```python
from build123d import *

# Parameters (mm, degrees)
F0_R     = 104
F0_R_2   = 68.5
F1_DEPTH = 19
F2_R     = 80
F2_R_2   = 74.5
F3_DEPTH = 14.1
F4_R     = 80
F5_DEPTH = 12
F6_SIZE2 = 1.1547005384
F6_SIZE  = 2
F7_R     = 5
F9_D     = 14
F9_DEPTH = 25.5
F9_TIP   = 4.2060243332


with BuildPart() as f1:
    # F0 (on Right) → F1 (new body)
    with BuildSketch(Plane.YZ):
        Circle(F0_R)
        Circle(F0_R_2, mode=Mode.SUBTRACT)
    extrude(amount=-F1_DEPTH)

    # F2 (on face) → F3 (join)
    with BuildSketch(Plane.YZ):
        Circle(F2_R)
        Circle(F2_R_2, mode=Mode.SUBTRACT)
    extrude(amount=F3_DEPTH)

    # F4 (on face) → F5 (cut)
    with BuildSketch(Plane(origin=(-19, 0, 0), x_dir=(0, -1, 0), z_dir=(-1, 0, 0))):
        Circle(F4_R)
    extrude(amount=-F5_DEPTH, mode=Mode.SUBTRACT)

    # F6
    f6_edges = [f1.edges().sort_by_distance(p)[0] for p in [
        (14.1, -80, 0),
    ]]
    f6_side = f1.faces().sort_by_distance((7.05, -80, 0))[0]
    chamfer(f6_edges, length=F6_SIZE, length2=F6_SIZE2, reference=f6_side)

    # F7
    f7_edges = [f1.edges().sort_by_distance(p)[0] for p in [
        (0, -74.5, 0),
    ]]
    fillet(f7_edges, radius=F7_R)

    # F9
    with Locations(Plane(origin=(-19, 0, 0), x_dir=(0, -1, 0), z_dir=(-1, 0, 0))):
        with Locations((0, -93), (-93, 0), (0, 93), (93, 0)):
            Hole(F9_D / 2, depth=F9_DEPTH)
            with Locations((0, 0, -(F9_DEPTH + F9_TIP / 2))):  # 118° drill point
                Cone(0, F9_D / 2, F9_TIP, mode=Mode.SUBTRACT)


solid = f1.part
```
Here's how the part is built. I have some questions about the finished solid (model axes, mm). A direction names the side the tool comes from. Coordinates: 2 decimals unless noted, no trailing zeros. Write each loop counter-clockwise with the first axis right and the second up, starting at its lowest first coordinate (ties: lowest second). Pieces come first, ordered by that corner, then holes. Notation, with made-up numbers: M 65,30.5 L 105,30.5 A24 ccw 105,44.5 Z; hole C -5.5,28.25 d4. An arc over 180 degrees is marked long. Answer as CSV lines item,"result". Start each with the question number.
Q1. Suppose I cut it at B-B, the plane z = 93. List the corners of the cut face in (x, y) for me.
Q2. I need wall thicknesses on probe 1 along Z at (x, y) = (-4.5, 0); probe 2 along X at (y, z) = (-86, 46); probe 3 along Y at (x, z) = (-7.5, -95). Which ranges of each line are inside material? Lowest first, please. Write a range as [from, to].
Q3. Suppose I cut it at C-C, the plane y = -88.5. List the corners of the cut face in (x, z) for me.
Q4. If we mould it in two halves opening along Y, with no side actions, what happens to faces 4 (the cylindrical face through (-13.08, 17.34, -78.1)), 5 (the cylindrical face through (-9.367, -82.531, -63.282)), 6 (the cylindrical face through (-9.37, -0.91, -86.06)), 7 (the flat face through (-19, -78, 24))? For each: pulls with the +Y half, pulls with the -Y half, needs draft (parallel to the pull), parting line crosses it, or undercut.
Q5. For faces 1 (the cylindrical face through (5.97, -17.34, -78.1)), 2 (the cylindrical face through (-3.451, 65.337, 20.576)), 3 (the flat face through (-7, -59, 36)), which set-ups out of +Z, -Z, +X, -X, +Y, -Y let a thin tool reach every point of the face, with its end or its side?
Q6. Suppose I cut it at D-D, the plane x = 2.5. List the corners of the cut face in (y, z) for me.
Q7. Will these pins go through, and if not, where does the flat tip stop? pin 1 Ø6 at (x, z) = (-8.5, 65.5) entering from -Y; pin 2 Ø10 at (x, y) = (10, 58) entering from -Z; pin 3 Ø5 at (y, z) = (55.5, -37) entering from +X.
Q8. Suppose I cut it at A-A, the plane y = 0. State how many separate pieces and enclosed holes the cut face has, then the cut area to 3 significant figures.
Entries:
1,outline,"M -19,-46.55 L 0,-46.55 L 0,-7 L -19,-7 Z; M -19,7 L 0,7 L 0,46.55 L -19,46.55 Z"
2,probe 1,"z = [-104, -100], [-86, -68.5], [68.5, 86], [100, 104]"
2,probe 2,"x = [-19, 0]"
2,probe 3,"y = [-42.32, -6.71], [6.71, 42.32]"
3,outline,"M -19,-54.62 L 0,-54.62 L 0,-5.36 L -19,-5.36 Z; M -19,5.36 L 0,5.36 L 0,54.62 L -19,54.62 Z"
4,face 4,"undercut"
4,face 5,"parting line crosses it"
4,face 6,"undercut"
4,face 7,"needs draft"
5,face 1,"+X"
5,face 2,"+X, -X"
5,face 3,"-X"
6,outline,"C 0,0 d160; hole C 0,0 d147.66"
7,pin 1,"stops at y = -83.12"
7,pin 2,"stops at z = -59.92"
7,pin 3,"stops at x = 0"
8,separate pieces,"4"
8,enclosed holes,"0"
8,area,"705 mm²"
